Geometry check sheet. Reference: the model listing, model coordinates, mm. A direction names the side the tool comes from. Round coordinates to 2 decimals unless told otherwise and drop trailing zeros. Loops run counter-clockwise (first coordinate to the right, second up) from the corner with the lowest first, then second, coordinate; pieces in that order, holes last.
```python
from build123d import *

# Parameters (mm, degrees)
BOSS_EXTRUDE1_DEPTH = 20
BOSS_EXTRUDE2_START = 20
BOSS_EXTRUDE2_DEPTH = 20
BOSS_EXTRUDE3_DEPTH = 3


with BuildPart() as part:
    # Sketch1 → Boss-Extrude1 (new body)
    with BuildSketch(Plane.XY):
        with BuildLine():
            Line((-39.43013831, -13.342220693), (-39.43013831, 19.556376021))
            ThreePointArc((-39.43013831, 19.556376021), (-34.879077983, 29.991705983), (-25.8204651, 36.88734186))
            Line((-25.8204651, 36.88734186), (-22.2204651, 36.88734186))
            Line((-22.2204651, 36.88734186), (-10.430426389, 32.607077664))
            Line((-10.430426389, 32.607077664), (11.569573611, 32.607077664))
            Line((11.569573611, 32.607077664), (23.359612322, 36.88734186))
            Line((23.359612322, 36.88734186), (26.959612322, 36.88734186))
            ThreePointArc((26.959612322, 36.88734186), (36.018225205, 29.991705983), (40.569285532, 19.556376021))
            Line((40.569285532, 19.556376021), (40.569285532, -13.342220693))
            ThreePointArc((40.569285532, -13.342220693), (23.896981794, -31.168666499), (0.569573611, -38.350581945))
            ThreePointArc((0.569573611, -38.350581945), (-22.757834572, -31.168666499), (-39.43013831, -13.342220693))
        make_face()
        with BuildLine():
            Line((-38.23013831, 19.556376021), (-38.23013831, -13.342220693))
            ThreePointArc((-38.23013831, -13.342220693), (-21.933714077, -29.946069187), (0.569573611, -35.850581945))
            ThreePointArc((0.569573611, -35.850581945), (23.072861298, -29.946069187), (39.369285532, -13.342220693))
            Line((39.369285532, -13.342220693), (39.369285532, 19.556376021))
            ThreePointArc((39.369285532, 19.556376021), (34.750379485, 28.298871636), (26.959612322, 34.38734186))
            Line((26.959612322, 34.38734186), (23.359612322, 34.38734186))
            Line((23.359612322, 34.38734186), (11.569573611, 30.107077664))
            Line((11.569573611, 30.107077664), (-10.430426389, 30.107077664))
            Line((-10.430426389, 30.107077664), (-22.2204651, 34.38734186))
            Line((-22.2204651, 34.38734186), (-25.8204651, 34.38734186))
            ThreePointArc((-25.8204651, 34.38734186), (-33.611232263, 28.298871636), (-38.23013831, 19.556376021))
        make_face(mode=Mode.SUBTRACT)
    extrude(amount=BOSS_EXTRUDE1_DEPTH)

    # Sketch2 → Boss-Extrude2 (add)
    with BuildSketch(Plane(origin=(0, 0, 0), x_dir=(-1, 0, 0), z_dir=(0, 0, -1)).offset(BOSS_EXTRUDE2_START)):
        with BuildLine():
            ThreePointArc((-26.959612322, 36.88734186), (-36.018225205, 29.991705983), (-40.569285532, 19.556376021))
            Line((-40.569285532, 19.556376021), (-39.369285532, 19.556376021))
            ThreePointArc((-39.369285532, 19.556376021), (-34.750379485, 28.298871636), (-26.959612322, 34.38734186))
            Line((-26.959612322, 34.38734186), (-23.359612322, 34.38734186))
            Line((-23.359612322, 34.38734186), (-11.569573611, 30.107077664))
            Line((-11.569573611, 30.107077664), (-0.569573611, 30.107077664))
            Line((-0.569573611, 30.107077664), (-0.569573611, 32.607077664))
            Line((-0.569573611, 32.607077664), (-11.569573611, 32.607077664))
            Line((-11.569573611, 32.607077664), (-23.359612322, 36.88734186))
            Line((-23.359612322, 36.88734186), (-26.959612322, 36.88734186))
        make_face()
        with BuildLine():
            Line((10.430426389, 32.607077664), (-0.569573611, 32.607077664))
            Line((-0.569573611, 32.607077664), (-0.569573611, 30.107077664))
            Line((-0.569573611, 30.107077664), (10.430426389, 30.107077664))
            Line((10.430426389, 30.107077664), (22.2204651, 34.38734186))
            Line((22.2204651, 34.38734186), (25.8204651, 34.38734186))
            ThreePointArc((25.8204651, 34.38734186), (33.611232263, 28.298871636), (38.23013831, 19.556376021))
            Line((38.23013831, 19.556376021), (39.43013831, 19.556376021))
            ThreePointArc((39.43013831, 19.556376021), (34.879077983, 29.991705983), (25.8204651, 36.88734186))
            Line((25.8204651, 36.88734186), (22.2204651, 36.88734186))
            Line((22.2204651, 36.88734186), (10.430426389, 32.607077664))
        make_face()
        with BuildLine():
            Line((-0.569573611, -38.350581945), (-0.569573611, -35.850581945))
            ThreePointArc((-0.569573611, -35.850581945), (-23.072861298, -29.946069187), (-39.369285532, -13.342220693))
            Line((-39.369285532, -13.342220693), (-40.569285532, -13.342220693))
            ThreePointArc((-40.569285532, -13.342220693), (-23.896981794, -31.168666499), (-0.569573611, -38.350581945))
        make_face()
        with BuildLine():
            Line((-0.569573611, -38.350581945), (-0.569573611, -35.850581945))
            ThreePointArc((-0.569573611, -35.850581945), (21.933714077, -29.946069187), (38.23013831, -13.342220693))
            Line((38.23013831, -13.342220693), (39.43013831, -13.342220693))
            ThreePointArc((39.43013831, -13.342220693), (22.757834572, -31.168666499), (-0.569573611, -38.350581945))
        make_face()
    extrude(amount=-BOSS_EXTRUDE2_DEPTH)

    # Sketch3 → Boss-Extrude3 (add)
    with BuildSketch(Plane.XY.offset(20)):
        with BuildLine():
            Line((-25.8204651, 36.88734186), (-22.2204651, 36.88734186))
            Line((-22.2204651, 36.88734186), (-10.430426389, 32.607077664))
            Line((-10.430426389, 32.607077664), (11.569573611, 32.607077664))
            Line((11.569573611, 32.607077664), (23.359612322, 36.88734186))
            Line((23.359612322, 36.88734186), (26.959612322, 36.88734186))
            ThreePointArc((26.959612322, 36.88734186), (36.018225205, 29.991705983), (40.569285532, 19.556376021))
            Line((40.569285532, 19.556376021), (40.569285532, -13.342220693))
            ThreePointArc((40.569285532, -13.342220693), (23.896981794, -31.168666499), (0.569573611, -38.350581945))
            ThreePointArc((0.569573611, -38.350581945), (-22.757834572, -31.168666499), (-39.43013831, -13.342220693))
            Line((-39.43013831, -13.342220693), (-39.43013831, 19.556376021))
            ThreePointArc((-39.43013831, 19.556376021), (-34.879077983, 29.991705983), (-25.8204651, 36.88734186))
        make_face()
    extrude(amount=BOSS_EXTRUDE3_DEPTH)


solid = part.part
```
1) Sectioned sample at C-C, the plane x = -11.5. Record the cut outline in (y, z).
Report:
outline: (-36.3, -20) - (-34.31, -20) - (-34.31, 20) - (30.5, 20) - (30.5, -20) - (33, -20) - (33, 23) - (-36.3, 23) - close
2) Sectioned sample at B-B, the plane y = 10.5. Record the cut outline in (x, z).
Report:
outline: (-39.43, 0) - (-38.23, 0) - (-38.23, 20) - (39.37, 20) - (39.37, 0) - (40.57, 0) - (40.57, 23) - (-39.43, 23) - close
3) Access from +Z, -Z, +X, -X, +Y, -Y to the whole of each face (thin tool, end or side, straight path). Record for faces 5 (the face through (17.382, 34.717, 1.199)), 6 (the face through (34.84, 28.19, -0.28)), 7 (the face through (1, 31, -20)).
Report:
face 5: +Z, -Z, +Y
face 6: -Z
face 7: -Z, +X, -X, +Y, -Y
4) Gauge pin test, flat ends, axial feed: pin 1 (4 mm diameter, centred on x = 25, z = -2, fed in from -Y); pin 2 (1 mm diameter, centred on x = 40, z = -5.5, fed in from -Y); pin 3 (3 mm diameter, centred on y = -24.5, z = -14, fed in from +X). Record the tip position at first contact, or that the pin passes through.
Report:
pin 1: stops at y = -31.72
pin 2: stops at y = -15.23
pin 3: stops at x = 33.72
5) Mould release check, pull along X, two halves, no side actions. Record for faces 1 (the face through (1, 30.107, 0)), 2 (the face through (35.918, 30.118, 1.199)), 3 (the face through (-22.22, -29.78, -0.28)), 4 (the face through (4, -36, -20)): +X half, -X half, draft (parallel to the pull), parting line (faces both ways), or undercut.
Report:
face 1: undercut
face 2: +X half
face 3: undercut
face 4: draft
6) Sectioned sample at D-D, the plane z = 3. Record the cut outline in (x, y), then the cut area to 3 significant figures.
Report:
outline: (-39.43, -13.34) arc R47.46 ccw to (0.57, -38.35) arc R47.46 ccw to (40.57, -13.34) - (40.57, 19.56) arc R22.61 ccw to (26.96, 36.89) - (23.36, 36.89) - (11.57, 32.61) - (-10.43, 32.61) - (-22.22, 36.89) - (-25.82, 36.89) arc R22.61 ccw to (-39.43, 19.56) - close; hole (-38.23, -13.34) arc R43.76 ccw to (0.57, -35.85) arc R43.76 ccw to (39.37, -13.34) - (39.37, 19.56) arc R23.64 ccw to (26.96, 34.39) - (23.36, 34.39) - (11.57, 30.11) - (-10.43, 30.11) - (-22.22, 34.39) - (-25.82, 34.39) arc R23.64 ccw to (-38.23, 19.56) - close
area: 446 mm2
7) Scan lines: line 1 along X through (y, z) = (-13, 9); line 2 along Z through (x, y) = (-6.5, -31); line 3 along Y through (x, z) = (-36, -1.5). Record each from-to range of solid material in increasing order.
Report:
line 1: x = -39.43 to -38.23, 39.37 to 40.57
line 2: z = 20 to 23
line 3: y = -18.81 to -16.94, 24.87 to 28.43
8) Sectioned sample at A-A, the plane z = -8. Record the cut outline in (x, y), then the cut area to 3 significant figures.
Report:
outline: (-39.43, -13.34) arc R47.46 ccw to (0.57, -38.35) arc R47.46 ccw to (40.57, -13.34) - (39.37, -13.34) arc R43.76 cw to (0.57, -35.85) arc R43.76 cw to (-38.23, -13.34) - close; (-39.43, 19.56) - (-38.23, 19.56) arc R23.64 cw to (-25.82, 34.39) - (-22.22, 34.39) - (-10.43, 30.11) - (11.57, 30.11) - (23.36, 34.39) - (26.96, 34.39) arc R23.64 cw to (39.37, 19.56) - (40.57, 19.56) arc R22.61 ccw to (26.96, 36.89) - (23.36, 36.89) - (11.57, 32.61) - (-10.43, 32.61) - (-22.22, 36.89) - (-25.82, 36.89) arc R22.61 ccw to start
area: 367 mm2
